Could you check a few things on this model? Use its own coordinates, in mm. Face numbers are marked on the shaded views. A direction names the side the tool comes from. Round coordinates to 2 decimals unless told otherwise and drop trailing zeros. Order: outer loops, then holes, each group sorted by start corner. A loop starts at its lowest first (then second) coordinate and runs counter-clockwise, first axis right, second up. Notation, with made-up numbers: (50, -16) - (56, -16) arc R23 ccw to (56, 7) - close; hole circle Ø3 at (54, -10.5). An arc over 180 degrees is marked (long way). Return JSON: item names as keys, results as strings. Group by question number.
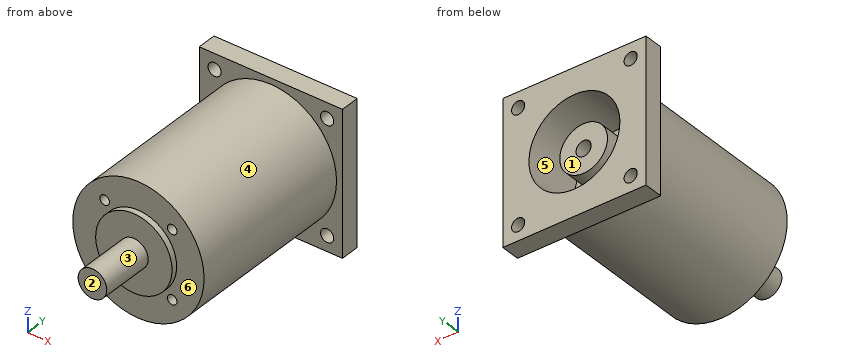
from build123d import *

# Parameters (mm, degrees)
SKETCH1_R           = 27.5
BOSS_EXTRUDE1_DEPTH = 72
SKETCH2_R           = 16
BOSS_EXTRUDE2_DEPTH = 2.5
SKETCH3_W           = 60
SKETCH3_H           = 60
BOSS_EXTRUDE3_DEPTH = 8
SKETCH4_R           = 6
BOSS_EXTRUDE4_DEPTH = 22.5
SKETCH5_R           = 2
CUT_EXTRUDE1_DEPTH  = 16
SKETCH6_R           = 19.05
CUT_EXTRUDE2_DEPTH  = 25
SKETCH7_R           = 10
SKETCH7_R_2         = 3.175
BOSS_EXTRUDE5_DEPTH = 20
SKETCH8_R           = 2.75
CUT_EXTRUDE3_DEPTH  = 10


with BuildPart() as part:
    # Sketch1 → Boss-Extrude1 (new body)
    with BuildSketch(Plane(origin=(0, 0, 0), x_dir=(1, 0, 0), z_dir=(0, 1, 0))):
        with Locations(Location((0, 0, 0), (0, 0, 270))):
            Circle(SKETCH1_R)
    extrude(amount=BOSS_EXTRUDE1_DEPTH)

    # Sketch2 → Boss-Extrude2 (add)
    with BuildSketch(Plane.XZ):
        with Locations(Location((0, 0, 0), (0, 0, 270))):
            Circle(SKETCH2_R)
    extrude(amount=BOSS_EXTRUDE2_DEPTH)

    # Sketch3 → Boss-Extrude3 (add)
    with BuildSketch(Plane(origin=(0, 72, 0), x_dir=(1, 0, 0), z_dir=(0, 1, 0))):
        Rectangle(SKETCH3_W, SKETCH3_H)
    extrude(amount=BOSS_EXTRUDE3_DEPTH)

    # Sketch4 → Boss-Extrude4 (add)
    with BuildSketch(Plane(origin=(0, -2.5, 0), x_dir=(-1, 0, 0), z_dir=(0, -1, 0))):
        with Locations(Location((0, 0, 0), (0, 0, 270))):
            Circle(SKETCH4_R)
    extrude(amount=BOSS_EXTRUDE4_DEPTH)

    # Sketch5 → Cut-Extrude1 (cut)
    with BuildSketch(Plane.XZ):
        with Locations(Location((14.142135624, 14.142135624, 0), (0, 0, 270))):
            Circle(SKETCH5_R)
        with Locations(Location((14.142135624, -14.142135624, 0), (0, 0, 270))):
            Circle(SKETCH5_R)
        with Locations(Location((-14.142135624, -14.142135624, 0), (0, 0, 270))):
            Circle(SKETCH5_R)
        with Locations(Location((-14.142135624, 14.142135624, 0), (0, 0, 270))):
            Circle(SKETCH5_R)
    extrude(amount=-CUT_EXTRUDE1_DEPTH, mode=Mode.SUBTRACT)

    # Sketch6 → Cut-Extrude2 (cut)
    with BuildSketch(Plane(origin=(0, 80, 0), x_dir=(1, 0, 0), z_dir=(0, 1, 0))):
        with Locations(Location((0, 0, 0), (0, 0, 270))):
            Circle(SKETCH6_R)
    extrude(amount=-CUT_EXTRUDE2_DEPTH, mode=Mode.SUBTRACT)

    # Sketch7 → Boss-Extrude5 (add)
    with BuildSketch(Plane(origin=(0, 55, 0), x_dir=(1, 0, 0), z_dir=(0, 1, 0))):
        with Locations(Location((0, 0, 0), (0, 0, 270))):
            Circle(SKETCH7_R)
        with Locations(Location((0, 0, 0), (0, 0, 270))):
            Circle(SKETCH7_R_2, mode=Mode.SUBTRACT)
    extrude(amount=BOSS_EXTRUDE5_DEPTH)

    # Sketch8 → Cut-Extrude3 (cut)
    with BuildSketch(Plane(origin=(0, 80, 0), x_dir=(1, 0, 0), z_dir=(0, 1, 0))):
        with Locations(Location((-23.571404551, 23.571404551, 0), (0, 0, 270))):
            Circle(SKETCH8_R)
        with Locations(Location((23.571404551, 23.571404551, 0), (0, 0, 270))):
            Circle(SKETCH8_R)
        with Locations(Location((23.571404551, -23.571404551, 0), (0, 0, 270))):
            Circle(SKETCH8_R)
        with Locations(Location((-23.571404551, -23.571404551, 0), (0, 0, 270))):
            Circle(SKETCH8_R)
    extrude(amount=-CUT_EXTRUDE3_DEPTH, mode=Mode.SUBTRACT)


solid = part.part
1) If I drill on line 1 along X through (y, z) = (60.25, 0) (3 decimals); line 2 along Y through (x, z) = (25.5, -26.5); line 3 along Y through (x, z) = (-15, -5), over which ranges is the centre line in solid material (lowest first)? Write a range as from..to.
2) I want a section at A-A, the plane y = 67. List the corners of the cut face in (x, z) for me (3 decimals), plus the area to 3 significant figures.
3) I want a section at B-B, the plane z = 0. List the corners of the cut face in (x, y) for me (3 decimals), plus the area to 3 significant figures.
4) For the marked faces 1, 2 and 3, which set-ups out of +Z, -Z, +X, -X, +Y, -Y let a thin tool reach every point of the face, with its end or its side?
5) Will these pins go through, and if not, where does the flat tip stop? pin 1 (1 mm diameter, centred on x = 15.5, z = 0.5, fed in from +Y); pin 2 (5 mm diameter, centred on x = 5.5, y = 24, fed in from +Z); pin 3 (1 mm diameter, centred on x = -4.5, z = 19, fed in from -Y).
6) We'd pull the mould along X, two halves only. Please class the marked faces 4, 5 and 6: +X half, -X half, draft (parallel to the pull), parting line (faces both ways), or undercut.
7) I want a section at C-C, the plane x = 0. List the corners of the cut face in (y, z) for me (3 decimals).
8) I want a section at D-D, the plane z = 22.5. List the corners of the cut face in (x, y) for me.
Outcome:
{
 "1": {"line 1": "-27.5..-19.05, -10..-3.175, 3.175..10, 19.05..27.5", "line 2": "72..80", "line 3": "-2.5..55"},
 "2": {"outline": "circle Ø55 at (0, 0); circle Ø20 at (0, 0); hole circle Ø38.1 at (0, 0); hole circle Ø6.35 at (0, 0)", "area": "1,520 mm^2"},
 "3": {"outline": "(-30, 72) - (-27.5, 72) - (-27.5, 0) - (-16, 0) - (-16, -2.5) - (-6, -2.5) - (-6, -25) - (6, -25) - (6, -2.5) - (16, -2.5) - (16, 0) - (27.5, 0) - (27.5, 72) - (30, 72) - (30, 80) - (19.05, 80) - (19.05, 55) - (10, 55) - (10, 75) - (3.175, 75) - (3.175, 55) - (-3.175, 55) - (-3.175, 75) - (-10, 75) - (-10, 55) - (-19.05, 55) - (-19.05, 80) - (-30, 80) - close", "area": "4,110 mm^2"},
 "4": {"face 1": "+Y", "face 2": "+Z, -Z, +X, -X, -Y", "face 3": "-Y"},
 "5": {"pin 1": "y = 55", "pin 2": "z = 27.34", "pin 3": "y = 0"},
 "6": {"face 4": "parting line", "face 5": "undercut", "face 6": "draft"},
 "7": {"outline": "(-25, -6) - (-2.5, -6) - (-2.5, -16) - (0, -16) - (0, -27.5) - (72, -27.5) - (72, -30) - (80, -30) - (80, -19.05) - (55, -19.05) - (55, -10) - (75, -10) - (75, -3.175) - (55, -3.175) - (55, 3.175) - (75, 3.175) - (75, 10) - (55, 10) - (55, 19.05) - (80, 19.05) - (80, 30) - (72, 30) - (72, 27.5) - (0, 27.5) - (0, 16) - (-2.5, 16) - (-2.5, 6) - (-25, 6) - close"},
 "8": {"outline": "(-30, 72) - (-26.1, 72) - (-26.1, 80) - (-30, 80) - close; (-21.04, 72) - (-15.81, 72) - (-15.81, 0) - (15.81, 0) - (15.81, 72) - (21.04, 72) - (21.04, 80) - (-21.04, 80) - close; (26.1, 72) - (30, 72) - (30, 80) - (26.1, 80) - close"}
}
